```python
from build123d import *

# Parameters (mm, degrees)
SKETCH1_R      = 1.50705101
SKETCH1_R_2    = 1.0795
SKETCH1_R_3    = 1.58353158
SKETCH1_W      = 32.345315457
SKETCH1_H      = 30
EXTRUDE1_DEPTH = 3.175


with BuildPart() as part:
    # Sketch1 → Extrude1 (new body)
    with BuildSketch(Plane(origin=(0, 0, 0), x_dir=(1, 0, 0), z_dir=(0, 1, 0))):
        Polygon((-67.158636898, 70.484310302), (-67.158636898, 74.492800404), (-68.408636898, 74.492800404), (-68.408636898, 76.742800404), (-67.158636898, 76.742800404), (-67.158636898, 85.234310302), (-81.279057464, 85.234310302), (-81.279057464, 91.584310302), (-91.279057464, 91.584310302), (-93.1320954, -13.415689698), (-83.1320954, -13.415689698), (-83.1320954, -7.065689698), (-67.402600688, -7.065689698), (-67.402600688, 1.425820201), (-68.652600688, 1.425820201), (-68.652600688, 3.675820201), (-67.402600688, 3.675820201), (-67.402600688, 7.684310302), (-64.502600688, 7.684310302), (-64.502600688, 3.675820201), (-63.252600688, 3.675820201), (-63.252600688, 1.425820201), (-64.502600688, 1.425820201), (-64.502600688, -7.065689698), (-3.311856943, -7.065689698), (-3.31328789, -13.417119454), (6.68671211, -13.417119454), (6.68671211, -7.065689698), (9.00171211, -7.065689698), (9.00171211, 1.771032224), (7.75171211, 1.771032224), (7.75171211, 4.021032224), (9.00171211, 4.021032224), (9.00171211, 7.684310302), (11.90171211, 7.684310302), (11.90171211, 4.021032224), (13.15171211, 4.021032224), (13.15171211, 1.771032224), (11.90171211, 1.771032224), (11.90171211, -7.065689698), (19.042987782, -7.065689698), (19.042987782, -13.417119454), (29.042987782, -13.417119454), (29.042987782, 91.482596586), (19.042987782, 91.482596586), (19.042987782, 85.132545763), (12.668135492, 85.132592736), (12.668135492, 76.295870815), (13.395675901, 76.295870815), (13.395675901, 74.045870815), (12.145675901, 74.045870815), (12.145675901, 70.382596586), (9.245675901, 70.382596586), (9.245675901, 74.045874665), (7.995675901, 74.045874665), (7.995675901, 76.295874665), (9.245675901, 76.295874665), (9.245675901, 85.132596586), (8.371396704, 85.132596586), (8.371396704, 91.482596586), (-1.628603296, 91.482596586), (-1.628603296, 85.132596586), (-64.258636898, 85.234310302), (-64.258636898, 76.742800404), (-63.008636898, 76.742800404), (-63.008636898, 74.492800404), (-64.258636898, 74.492800404), (-64.258636898, 70.484310302), align=None)
        with Locations(Location((-78.42302428, 17.147481819, 0), (0, 0, 270))):
            Circle(SKETCH1_R, mode=Mode.SUBTRACT)
        with Locations(Location((-27.62307508, 32.387481819, 0), (0, 0, 270))):
            Circle(SKETCH1_R_2, mode=Mode.SUBTRACT)
        with Locations(Location((-27.62307508, 60.327481819, 0), (0, 0, 270))):
            Circle(SKETCH1_R_3, mode=Mode.SUBTRACT)
        with Locations((-5.646064502, 40.784310302)):
            Rectangle(SKETCH1_W, SKETCH1_H, mode=Mode.SUBTRACT)
    extrude(amount=EXTRUDE1_DEPTH)


solid = part.part
```
Source: CAD feature listing. Evaluate the final solid. Frame: model axes, mm. A direction names the side the tool comes from. Coordinates: 2 decimals unless noted, no trailing zeros. Write each loop counter-clockwise with the first axis right and the second up, starting at its lowest first coordinate (ties: lowest second). Pieces come first, ordered by that corner, then holes. Notation, with made-up numbers: M 38.5,14 L 62.5,14 A21 cw 62.5,35 Z; hole C 86,-2.75 d8. An arc over 180 degrees is marked long. Answer as a JSON object with one key per item and string values.
1. Cut plane B-B on x = -7. Output: boundary loops of the cut face in (y, z) (3 decimals), plus the area to 3 significant figures.
Evaluation:
{"outline": "M 0,-85.141 L 3.175,-85.141 L 3.175,-55.784 L 0,-55.784 Z; M 0,-25.784 L 3.175,-25.784 L 3.175,7.066 L 0,7.066 Z", "area": "198 mm^2"}
2. Ray query, L1, parallel to Z at x = -16.5, y = 2.1; L2, parallel to Z at x = -4, y = 2.65; L3, parallel to Z at x = -83, y = 3.05. Return the intervals inside material, ascending.
Evaluation:
{"L1": "-85.16 to -55.78, -25.78 to 7.07", "L2": "-85.14 to -55.78, -25.78 to 7.07", "L3": "-91.58 to 7.07"}
3. Cut plane D-D on y = 0.8. State how many separate pieces and enclosed holes the cut face has, plus the area to 3 significant figures.
Evaluation:
{"separate pieces": "1", "enclosed holes": "4", "area": "10,400 mm^2"}
4. Access query for faces 1 (the flat face through (-21.819, 2, -41)), 2 (the flat face through (19.043, 2, -88)), 3 (the flat face through (-66, 2, -7.684)). Directions: +Z, -Z, +X, -X, +Y, -Y. A direction counts if a zero-diameter tool reaches every point of the face in a straight line with its end or side. Return the directions, or none.
Evaluation:
{"face 1": "+Y, -Y", "face 2": "-Z, +Y, -Y", "face 3": "+Z, +Y, -Y"}
5. Draft query along X for faces 4 (the flat face through (-1.629, 2, -88)), 5 (the flat face through (3, 2, -91.483)). Return one class per face: released by +X, released by -X, zero draft, split by the parting line, or undercut.
Evaluation:
{"face 4": "undercut", "face 5": "zero draft"}
6. Contact query for flat-ended pins moving along their axis: P1, Ø1, axis at y = 1, z = -6, coming from the -X side; P2, Ø1.4, axis at x = 8.5, y = 2, coming from the +Z side; P3, Ø0.6, axis at x = 12.5, y = 1, coming from the -Z side. Output: stop coordinate, or through.
Evaluation:
{"P1": "x = -92.8", "P2": "z = 7.07", "P3": "z = -85.13"}
7. Cut plane C-C on z = -37. Output: boundary loops of the cut face in (x, y) (3 decimals), plus the area to 3 significant figures.
Evaluation:
{"outline": "M -92.242,0 L -21.819,0 L -21.819,3.175 L -92.242,3.175 Z; M 10.527,0 L 29.043,0 L 29.043,3.175 L 10.527,3.175 Z", "area": "282 mm^2"}
8. Cut plane A-A on z = -78.5. Output: boundary loops of the cut face in (x, y) (3 decimals).
Evaluation:
{"outline": "M -91.51,0 L -67.159,0 L -67.159,3.175 L -91.51,3.175 Z; M -64.259,0 L 9.246,0 L 9.246,3.175 L -64.259,3.175 Z; M 12.668,0 L 29.043,0 L 29.043,3.175 L 12.668,3.175 Z"}
